Design review of the part built by this model. Coordinates are the model's own, in mm. Face numbers are marked on the shaded views. Give positions to 0.01 mm unless a question says otherwise; leave off trailing zeros. Order: outer loops, then holes, each group sorted by start corner. A loop starts at its lowest first (then second) coordinate and runs counter-clockwise, first axis right, second up. Notation, with made-up numbers: M 78.25,55.5 L 100.25,55.5 A15 ccw 100.25,60.5 Z; hole C -34,37 d9. An arc over 180 degrees is marked long. Answer as a JSON object with one key per item and string values.
from build123d import *

# Parameters (mm, degrees)
F0_R     = 10.75
F0_R_2   = 8.75
F1_DEPTH = 100
F2_R     = 2.5
F3_DEPTH = 25


with BuildPart() as f1:
    # F0 (on Front) → F1 (new body)
    with BuildSketch(Plane.XZ):
        Circle(F0_R)
        Circle(F0_R_2, mode=Mode.SUBTRACT)
    extrude(amount=F1_DEPTH)

    # F2 (on Top) → F3 (cut, symmetric)
    with BuildSketch(Plane.XY):
        with Locations((0, -5)):
            Circle(F2_R)
        with Locations((0, -39)):
            Circle(F2_R)
    extrude(amount=F3_DEPTH, both=True, mode=Mode.SUBTRACT)


solid = f1.part
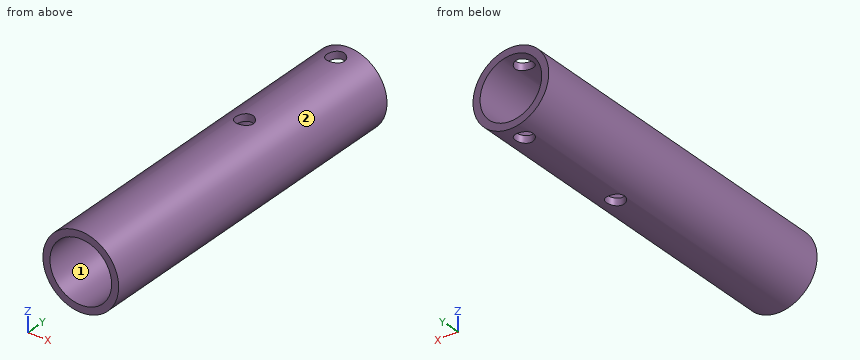
(1) To check wall thickness, follow L1, parallel to Y at x = 0, z = 10.05; L2, parallel to Z at x = 0, y = -33; L3, parallel to X at y = -39, z = -9.9. State the ranges of each line that lie inside material, in increasing order. Write a range as from..to.
Checked values:
{"L1": "y = -100..-41.5, -36.5..-7.5, -2.5..0", "L2": "z = -10.75..-8.75, 8.75..10.75", "L3": "x = -4.19..-2.5, 2.5..4.19"}
(2) We need section C-C (y = -39). Write out the cut boundary in (x, z).
Checked values:
{"outline": "M -2.5,-10.46 L -2.5,-8.39 A8.75 cw -2.5,8.39 L -2.5,10.46 A10.75 ccw Z; M 2.5,-10.46 A10.75 ccw 2.5,10.46 L 2.5,8.39 A8.75 cw 2.5,-8.39 Z"}
(3) We need section A-A (z = 0). Write out the cut boundary in (x, y).
Checked values:
{"outline": "M -10.75,-100 L -8.75,-100 L -8.75,0 L -10.75,0 Z; M 8.75,-100 L 10.75,-100 L 10.75,0 L 8.75,0 Z"}
(4) Insertion check: pin 1 (6 mm diameter, centred on y = -46, z = -4, fed in from +X); pin 2 (8 mm diameter, centred on x = 5.5, y = -68, fed in from -Z); pin 3 (1.5 mm diameter, centred on y = -11, z = -1.5, fed in from -X). Each pin has a flat end and moves straight along its axis. Give the tip position at first contact, or say it passes through.
Checked values:
{"pin 1": "stops at x = 10.7", "pin 2": "stops at z = -10.64", "pin 3": "stops at x = -10.72"}
(5) We need section D-D (y = -67). Write out the cut boundary in (x, z), plus the area to 3 significant figures.
Checked values:
{"outline": "C 0,0 d21.5; hole C 0,0 d17.5", "area": "123 mm^2"}
(6) We need section B-B (x = 0.75). Write out the cut boundary in (y, z), plus the area to 3 significant figures.
Checked values:
{"outline": "M -100,-10.72 L -41.38,-10.72 L -41.38,-8.72 L -100,-8.72 Z; M -100,8.72 L -41.38,8.72 L -41.38,10.72 L -100,10.72 Z; M -36.62,-10.72 L -7.38,-10.72 L -7.38,-8.72 L -36.62,-8.72 Z; M -36.62,8.72 L -7.38,8.72 L -7.38,10.72 L -36.62,10.72 Z; M -2.62,-10.72 L 0,-10.72 L 0,-8.72 L -2.62,-8.72 Z; M -2.62,8.72 L 0,8.72 L 0,10.72 L -2.62,10.72 Z", "area": "363 mm^2"}
(7) Draft analysis for pull direction X (two halves, no side actions). For the marked faces 1 and 2, state which applies: +X half, -X half, draft (parallel to the pull), parting line (faces both ways), or undercut.
Checked values:
{"face 1": "undercut", "face 2": "parting line"}
